Geometry: see drawing. Coordinates: mm, zero at the bounding-box minimum. A direction names the side the tool comes from. Round coordinates to 2 decimals unless told otherwise and drop trailing zeros. Write each loop counter-clockwise with the first axis right and the second up, starting at its lowest first coordinate (ties: lowest second). Pieces come first, ordered by that corner, then holes. Notation, with made-up numbers: M 58.25,-36 L 73.25,-36 A17 ccw 73.25,-31 Z; hole C -4.5,83.25 d5. An arc over 180 degrees is marked long. Use one line per item in the form item = value. Start each with the question number.
Item 1: Reachability of the marked faces 4, 5 and 6 from +Z, -Z, +X, -X, +Y, -Y: full face, straight path, thin tool, end or side. Return the list, or none.
Item 2: Section query D-D (x = 3.25). Return loops of the section in (y, z).
Item 3: Ray query, probe 1 along Z at (x, y) = (12, 13.75) (1 decimal); probe 2 along Y at (x, z) = (19.25, 17.5); probe 3 along Z at (x, y) = (9.5, 16.25) (1 decimal). Return the intervals inside material, ascending.
Item 4: Pin query (flat end, axial travel): pin 1 Ø1 at (y, z) = (13, 19) entering from -X (1 decimal); pin 2 Ø2 at (y, z) = (18.5, 5) entering from -X; pin 3 Ø3.5 at (x, y) = (12, 8) entering from -Z; pin 4 Ø5.5 at (x, z) = (11.91, 11.91) entering from -Y. Return the tip coordinate at first contact, or that it passes through.
Item 5: Section query C-C (z = 9). Return loops of the section in (x, y) (1 decimal).
Item 6: Section query B-B (x = 15). Return loops of the section in (y, z) (1 decimal), and give its area (3 significant figures).
Item 7: Section query A-A (y = 15.75). Return loops of the section in (x, z) (1 decimal).
Item 8: Pull-direction query (X, two-part tool) for the marked faces 1, 2 and 3; classes: pulls with the +X half, pulls with the -X half, needs draft (parallel to the pull), parting line crosses it, or undercut.
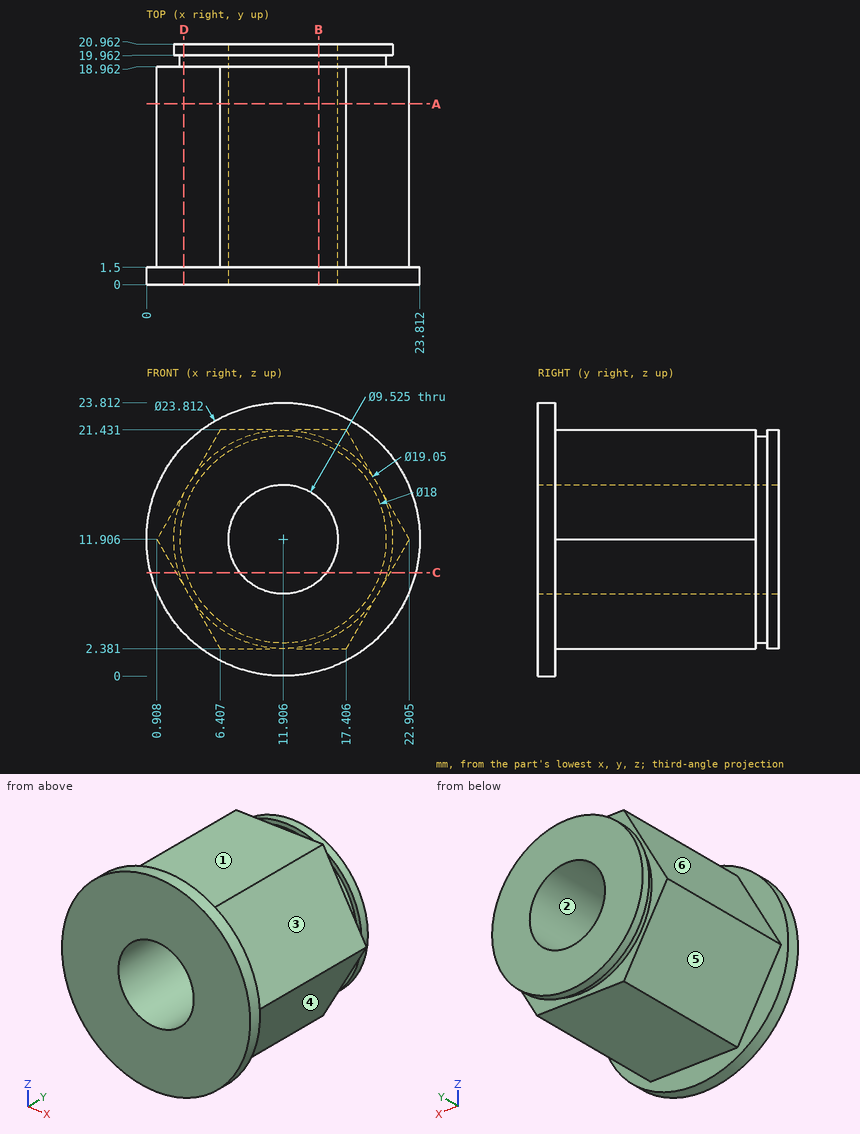
Working result:
q1.face_4 = -Z, +X, +Y
q1.face_5 = -Z, -X, +Y
q1.face_6 = +Z, -X, +Y
q2.outline = M 0,3.73 L 1.5,3.73 L 1.5,7.85 L 18.96,7.85 L 18.96,9.44 L 19.96,9.44 L 19.96,7.93 L 20.96,7.93 L 20.96,15.88 L 19.96,15.88 L 19.96,14.37 L 18.96,14.37 L 18.96,15.96 L 1.5,15.96 L 1.5,20.08 L 0,20.08 Z
q3.probe_1 = 2.4 to 7.1, 16.7 to 21.4
q3.probe_2 = 0 to 18.96, 19.96 to 20.96
q3.probe_3 = 2.4 to 7.8, 16 to 21.4
q4.pin_1 = 4.7
q4.pin_2 = 4.32
q4.pin_3 = 2.38
q4.pin_4 = through
q5.outline = M 0.4,0 L 8.1,0 L 8.1,21 L 2.8,21 L 2.8,20 L 3.4,20 L 3.4,19 L 2.6,19 L 2.6,1.5 L 0.4,1.5 Z; M 15.7,0 L 23.5,0 L 23.5,1.5 L 21.2,1.5 L 21.2,19 L 20.4,19 L 20.4,20 L 21,20 L 21,21 L 15.7,21 Z
q6.outline = M 0,0.4 L 1.5,0.4 L 1.5,2.4 L 19,2.4 L 19,3.5 L 20,3.5 L 20,2.9 L 21,2.9 L 21,8.3 L 0,8.3 Z; M 0,15.5 L 21,15.5 L 21,20.9 L 20,20.9 L 20,20.4 L 19,20.4 L 19,21.4 L 1.5,21.4 L 1.5,23.4 L 0,23.4 Z
q6.area = 250 mm²
q7.outline = M 0.9,11.9 L 6.4,2.4 L 17.4,2.4 L 22.9,11.9 L 17.4,21.4 L 6.4,21.4 Z; hole C 11.9,11.9 d9.5
q8.face_1 = needs draft
q8.face_2 = undercut
q8.face_3 = pulls with the +X half
